Check sheet for the modelled part. Datum: model origin and axes. Units: mm. Face numbers are marked on the shaded views. A direction names the side the tool comes from. Give positions to 0.01 mm unless a question says otherwise; leave off trailing zeros. Write each loop counter-clockwise with the first axis right and the second up, starting at its lowest first coordinate (ties: lowest second). Pieces come first, ordered by that corner, then holes. Notation, with made-up numbers: (33.5, 49) -> (89.5, 49) arc R10 cw to (89.5, 62) -> close; hole circle Ø7 at (-29, -31). An arc over 180 degrees is marked (long way). Return JSON: item names as keys, results as strings.
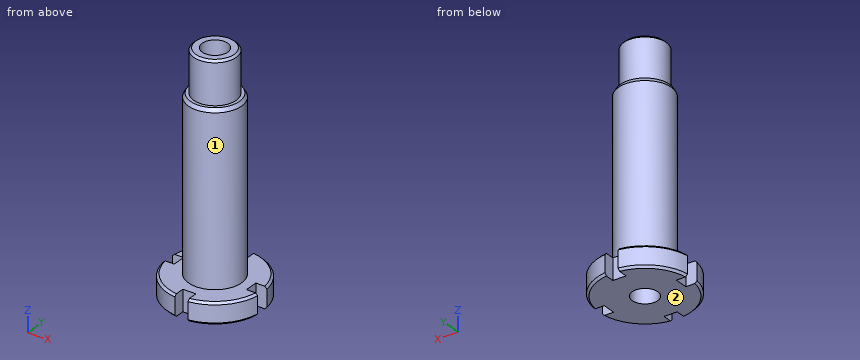
from build123d import *

# Parameters (mm, degrees)
CHANFREIN1_SIZE              = 1
ESQUISSE3_R                  = 6
ENL_V_MAT_EXTRU_2_DEPTH      = 111
ENL_V_MAT_EXTRU_1_DEPTH      = 111
R_P_TITION_CIRCULAIRE1_COUNT = 4
CHANFREIN2_SIZE              = 1
CHANFREIN2_SIZE2             = 1.732050808


with BuildPart() as part:
    # Esquisse1 → Révolution1 (revolve)
    with BuildSketch(Plane(origin=(0, 0, 0), x_dir=(0, 0, -1), z_dir=(1, 0, 0)), mode=Mode.PRIVATE) as r_volution1_sk:
        Polygon((-110, 0), (-110, 10), (-90, 10), (-90, 12.5), (-10, 12.5), (-10, 22.5), (0, 22.5), (0, 0), align=None)
    revolve(r_volution1_sk.sketch.rotate(Axis((0, 0, 0), (0, 0, 1)), 90), axis=Axis((0, 0, 0), (0, 0, 1)))  # turned: the seam where the file's is

    # Chanfrein1
    chanfrein1_edges = [part.edges().sort_by_distance(p)[0] for p in [
        (22.5, 0, 0),
        (22.5, 0, 10),
        (10, 0, 110),
    ]]
    chamfer(chanfrein1_edges, length=CHANFREIN1_SIZE)

    # Esquisse3 → Enlèv. mat.-Extru.2 (cut, through all)
    with BuildSketch(Plane(origin=(0, 0, 0), x_dir=(-1, 0, 0), z_dir=(0, 0, -1))):
        Circle(ESQUISSE3_R)
    extrude(amount=-ENL_V_MAT_EXTRU_2_DEPTH, mode=Mode.SUBTRACT)

    # Esquisse2 → Enlèv. mat.-Extru.1 (cut, through all)
    with BuildSketch(Plane(origin=(0, 0, 0), x_dir=(-1, 0, 0), z_dir=(0, 0, -1))):
        with BuildLine():
            Line((-3.1, 22.285421243), (-3.1, 17))
            Line((-3.1, 17), (3.1, 17))
            Line((3.1, 17), (3.1, 22.285421243))
            ThreePointArc((3.1, 22.285421243), (0, 22.5), (-3.1, 22.285421243))
        make_face()
    enl_v_mat_extru_1 = extrude(amount=-ENL_V_MAT_EXTRU_1_DEPTH, mode=Mode.SUBTRACT)

    # Répétition circulaire1: Enlèv. mat.-Extru.1 ×4 about axis
    r_p_tition_circulaire1_axis = Axis((0, 0, 0), (0, 0, 1))
    for i in range(1, R_P_TITION_CIRCULAIRE1_COUNT):
        add(enl_v_mat_extru_1.rotate(r_p_tition_circulaire1_axis, i * 360 / R_P_TITION_CIRCULAIRE1_COUNT), mode=Mode.SUBTRACT)

    # Chanfrein2
    chanfrein2_edges = [part.edges().sort_by_distance(p)[0] for p in [
        (12.5, 0, 90),
    ]]
    chanfrein2_side = [part.faces().sort_by_distance(p)[0] for p in [
        (10.353553391, 0, 90),
    ]]
    chamfer(chanfrein2_edges, length=CHANFREIN2_SIZE, length2=CHANFREIN2_SIZE2, reference=chanfrein2_side[0])


solid = part.part
(1) Cross-section at A-A on x = 0. Enter the section's corners in (y, z).
Reply:
{"outline": "(-17, 0) -> (-6, 0) -> (-6, 110) -> (-9, 110) -> (-10, 109) -> (-10, 90) -> (-11.5, 90) -> (-12.5, 88.27) -> (-12.5, 10) -> (-17, 10) -> close; (6, 0) -> (17, 0) -> (17, 10) -> (12.5, 10) -> (12.5, 88.27) -> (11.5, 90) -> (10, 90) -> (10, 109) -> (9, 110) -> (6, 110) -> close"}
(2) Cross-section at D-D on z = 14.5. Enter the section's corners in (x, y).
Reply:
{"outline": "circle Ø25 at (0, 0); hole circle Ø12 at (0, 0)"}
(3) Depth check by flat-ended pin: pin 1 Ø3 at (x, z) = (0, 6) entering from +Y; pin 2 Ø8 at (y, z) = (-9.5, 95.5) entering from +X; pin 3 Ø6 at (x, z) = (-19, 5.5) entering from -Y; pin 4 Ø10 at (x, y) = (-16, 1) entering from -Z. Enter the tip coordinate at first touch or a pass-through.
Reply:
{"pin 1": "y = 17", "pin 2": "x = 8.35", "pin 3": "y = -15.82", "pin 4": "z = 0"}
(4) Thickness scan on L1, parallel to Y at x = 0, z = 33; L2, parallel to Z at x = 12.5, y = -2.5; L3, parallel to X at y = -5, z = 63.5. Record the ranges inside material, lowest first.
Reply:
{"L1": "-12.5 to -6, 6 to 12.5", "L2": "0 to 10", "L3": "-11.46 to -3.32, 3.32 to 11.46"}
(5) Cross-section at C-C on z = 92. Enter the section's corners in (x, y).
Reply:
{"outline": "circle Ø20 at (0, 0); hole circle Ø12 at (0, 0)"}
(6) Set-up check for the marked faces 1 and 2: record each of +Z, -Z, +X, -X, +Y, -Y from which the full face is reachable in a straight line by a thin tool's end or side.
Reply:
{"face 1": "+Z", "face 2": "-Z, +X, -X, +Y, -Y"}
